Autodesk Inventor part; units mm, degrees
ref_plane "YZ Plane" through (0, 0, 0) normal (1, 0, 0) x (0, 1, 0)
ref_plane "XZ Plane" through (0, 0, 0) normal (0, 1, 0) x (-1, 0, 0)
ref_plane "XY Plane" through (0, 0, 0) normal (0, 0, 1) x (1, 0, 0)
sketch "Szkic1" plane through (0, 0, 0) normal (0, 1, 0) x (-1, 0, 0)
  line L0 (10, 0) -> (0, 0)
  line L1 (0, 0) -> (0, -25)
  line L2 (0, -25) -> (10, -25)
  line L3 (10, -25) -> (10, 0)
  dimension "d0" = 25
  dimension "d1" = 10
  dimension "d13" = 0
  dimension "d14" = 0
extrude "Płyta1" add sketch "Szkic1" along normal blind 2
sketch "Szkic2" plane through (-10, 0, -23) normal (0, 0, -1) x (-1, 0, 0)
  line L0 (-10, 0) -> (0, 0)
  line L1 (0, 0) -> (0, 15.5)
  line L2 (0, 15.5) -> (-10, 15.5)
  line L3 (-10, 15.5) -> (-10, 0)
edge flange "Kołnierz1" height 15.5 angle 90 thickness 2 bend radius 2 thickness toward (0, 0, -1) relief tear relief width 2 relief depth 1 edges at (-5, 2, -25) wall of the first edge with corners at (0, 0, -23) (-10, 0, -23) (-10, 15.5, -23) (0, 15.5, -23)
bend "Zagięcie1"
corner "Narożnik1"
sketch "Szkic4" plane through (0, 2, 0) normal (0, 1, 0) x (1, 0, 0)
  line L0 (-10, 0) -> (-10, 21)
  line L1 (0, 0) -> (-10, 0)
  point P0 (-5, 5)
  point P1 (-5, 12)
  dimension "d48" = 5
  dimension "d49" = 7
sketch "Szkic5" plane through (-10, 15.5, -23) normal (0, 0, 1) x (1, 0, 0)
  line L0 (10, 0) -> (0, 0)
  line L1 (0, 0) -> (0, -11.5)
  point P0 (10, -15.5)
  point P1 (5, -8.5)
  point P2 (5, -2.5)
  dimension "d50" = 6
  dimension "d51" = 2.5
hole "Otwór1" at (-5, 7, -23) at (-5, 13, -23) direction (0, 0, -1) diameter 2.9 end through all
hole "Otwór2" at (-5, 2, -5) at (-5, 2, -12) direction (0, -1, 0) diameter 4.22 end through all
chamfer "Faza1" distance 0.1 angle 45 2 edges at (-5, 2, -7.11) (-5, 2, -14.11)
equation "\"d36\" = Grubość"
equation "\"d43\" = Grubość"
equation "\"d2\" = Grubość"
equation "\"d3\" = SzerokośćGięciaPodcięcia"
equation "\"d4\" = GłębokośćGięciaPodcięcia"
equation "\"d5\" = MinimalnaPozostałość"
equation "\"d6\" = PromieńPrzejścia"
equation "\"d9\" = PromieńGięcia"
equation "\"d10\" = RozmiarPodcięciaNarożnika"
equation "\"d11\" = Wielk_odstępu"
equation "\"d12\" = Rozmiar_promienia_Jacobiego"
equation "\"PromieńGięcia\" = Grubość"
equation "\"SzerokośćGięciaPodcięcia\" = Grubość"
equation "\"GłębokośćGięciaPodcięcia\" = 0.5 * Grubość"
equation "\"RozmiarPodcięciaNarożnika\" = 4 * Grubość"
equation "\"MinimalnaPozostałość\" = 2 * Grubość"
equation "\"PromieńPrzejścia\" = PromieńGięcia"
equation "\"Rozmiar_promienia_Jacobiego\" = PromieńGięcia"
equation "\"Wielk_odstępu\" = Grubość"
properties material "Aluminium 6061"
Here's how the part is built. I have some questions about the finished solid (model axes, mm). A direction names the side the tool comes from. Coordinates: 2 decimals unless noted, no trailing zeros. Loops run counter-clockwise (first coordinate to the right, second up) from the corner with the lowest first, then second, coordinate; pieces in that order, holes last.
1. Imagine slicing it at D-D, the plane x = -1.5. Please give me the cut outline in (y, z), and give its area (3 significant figures).
2. Imagine slicing it at C-C, the plane x = -5. Please give me the cut outline in (y, z).
3. For faces 1 (the flat face through (-5, 10, -23)), 2 (the cylindrical face through (-5.07, 1.203, -23.859)), which set-ups out of +Z, -Z, +X, -X, +Y, -Y let a thin tool reach every point of the face, with its end or its side?
4. I need wall thicknesses on L1, parallel to X at y = 7, z = -23.95; L2, parallel to X at y = 0.5, z = -12; L3, parallel to Z at x = -5, y = 0.5. Which ranges of each line are inside material? Lowest first, please.
5. Imagine slicing it at A-A, the plane y = 13. Please give me the cut outline in (x, z).
6. If we mould it in two halves opening along X, with no side actions, what happens to faces 3 (the cylindrical face through (-4.12, 14.15, -24.01)), 4 (the flat face through (-5, 15.5, -24)), 5 (the flat face through (0, 1, -16))? For each: pulls with the +X half, pulls with the -X half, needs draft (parallel to the pull), parting line crosses it, or undercut.
7. Imagine slicing it at B-B, the plane z = -5. Please give me the cut outline in (x, y).
8. For P1, Ø3, axis at x = -6, y = 8, coming from the +Z side; P2, Ø4, axis at x = -5, z = -12, coming from the -Y side; P3, Ø2, axis at x = -8, y = 4, coming from the +Z side, each with a flat end and sliding along its axis, tell me the tip position at first contact or that it passes through.
Taken from the geometry:
1. outline: (0, -21) arc R4 ccw to (4, -25) - (15.5, -25) - (15.5, -23) - (4, -23) arc R2 cw to (2, -21) - (2, 0) - (0, 0) - close
1. area: 74.4 mm2
2. outline: (0, -21) arc R4 ccw to (4, -25) - (5.55, -25) - (5.55, -23) - (4, -23) arc R2 cw to (2, -21) - (2, -14.21) - (1.9, -14.11) - (0, -14.11) - close; (0, -9.89) - (1.9, -9.89) - (2, -9.79) - (2, -7.21) - (1.9, -7.11) - (0, -7.11) - close; (0, -2.89) - (1.9, -2.89) - (2, -2.79) - (2, 0) - (0, 0) - close; (8.45, -25) - (11.55, -25) - (11.55, -23) - (8.45, -23) - close; (14.45, -25) - (15.5, -25) - (15.5, -23) - (14.45, -23) - close
3. face 1: +Z, +X, -X, +Y
3. face 2: -Z, +X, -X, -Y
4. L1: x = -10 to -6.45, -3.55 to 0
4. L2: x = -10 to -7.11, -2.89 to 0
4. L3: z = -22.94 to -14.11, -9.89 to -7.11, -2.89 to 0
5. outline: (-10, -25) - (-6.45, -25) - (-6.45, -23) - (-10, -23) - close; (-3.55, -25) - (0, -25) - (0, -23) - (-3.55, -23) - close
6. face 3: undercut
6. face 4: needs draft
6. face 5: pulls with the +X half
7. outline: (-10, 0) - (-7.11, 0) - (-7.11, 1.9) - (-7.21, 2) - (-10, 2) - close; (-2.89, 0) - (0, 0) - (0, 2) - (-2.79, 2) - (-2.89, 1.9) - close
8. P1: stops at z = -23
8. P2: passes through
8. P3: stops at z = -22.73
